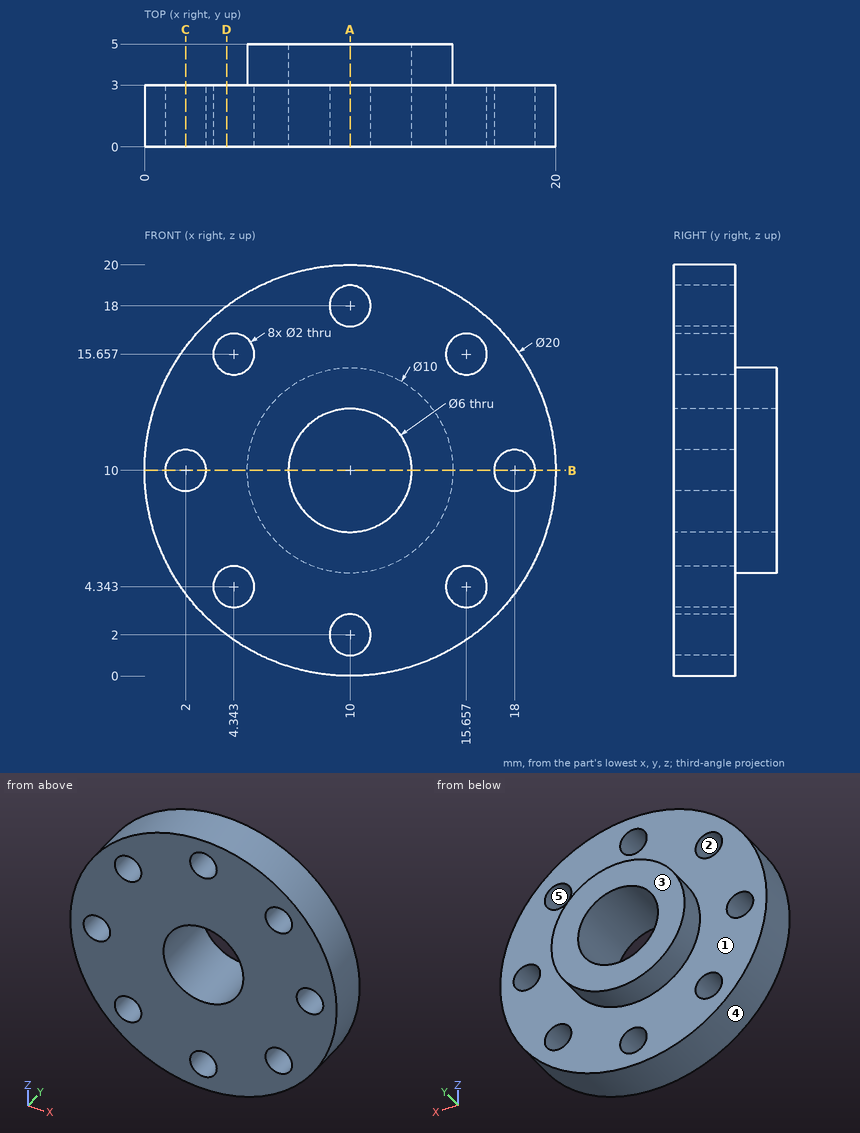
Print and shaded views of the part. All mm, measured from the part's lowest x, y and z. A direction names the side the tool comes from. Coordinates: 2 decimals unless noted, no trailing zeros. Loops run counter-clockwise (first coordinate to the right, second up) from the corner with the lowest first, then second, coordinate; pieces in that order, holes last. Notation, with made-up numbers: (4, -12) - (49, -12) arc R24 cw to (49, 14) - close; hole circle Ø1 at (-24.5, -3). An arc over 180 degrees is marked (long way). Use one line per item in the form item = value. Start each with the question number.
1) Band-saw the part on B-B (z = 10). Give the cut face in (x, y).
2) Drill centre lines: L1, parallel to Z at x = 10, y = 4.15; L2, parallel to X at y = 2.4, z = 5; L3, parallel to Z at x = 10, y = 1. Where is each one in solid material? Low to high. Write a range as from..to.
3) Tool access for the marked faces 1 and 2: list every direction of +Z, -Z, +X, -X, +Y, -Y with a clear straight run to the whole face (end or side of a thin tool).
4) Band-saw the part on D-D (x = 4). Give the cut face in (y, z), and give its area (3 significant figures).
5) Two-plate mould, pull along Z, no slides. Class the marked faces 3, 4 and 5: +Z half, -Z half, draft (parallel to the pull), parting line (faces both ways), or undercut.
6) Flat gauge pins, fed straight in: pin 1 (4 mm diameter, centred on x = 16.5, z = 6, fed in from +Y); pin 2 (3 mm diameter, centred on x = 13, y = 2, fed in from -Z); pin 3 (3 mm diameter, centred on y = 1.5, z = 18, fed in from -X). Where does each tip first touch, or does it go through?
7) Band-saw the part on C-C (x = 2). Give the cut face in (y, z).
8) Band-saw the part on A-A (x = 10). Give the cut face in (y, z), and give its area (3 significant figures).
Check values:
q1.outline = (0, 0) - (1, 0) - (1, 3) - (0, 3) - close; (3, 0) - (7, 0) - (7, 5) - (5, 5) - (5, 3) - (3, 3) - close; (13, 0) - (17, 0) - (17, 3) - (15, 3) - (15, 5) - (13, 5) - close; (19, 0) - (20, 0) - (20, 3) - (19, 3) - close
q2.L1 = 5..7, 13..15
q2.L2 = 1.34..3.59, 5.1..14.9, 16.41..18.66
q2.L3 = 0..1, 3..7, 13..17, 19..20
q3.face_1 = +Y
q3.face_2 = +Y, -Y
q4.outline = (0, 2) - (3, 2) - (3, 3.4) - (0, 3.4) - close; (0, 5.28) - (3, 5.28) - (3, 14.72) - (0, 14.72) - close; (0, 16.6) - (3, 16.6) - (3, 18) - (0, 18) - close
q4.area = 36.7 mm2
q5.face_3 = draft
q5.face_4 = parting line
q5.face_5 = undercut
q6.pin_1 = 3
q6.pin_2 = 0.11
q6.pin_3 = 2.4
q7.outline = (0, 4) - (3, 4) - (3, 9) - (0, 9) - close; (0, 11) - (3, 11) - (3, 16) - (0, 16) - close
q8.outline = (0, 0) - (3, 0) - (3, 1) - (0, 1) - close; (0, 3) - (3, 3) - (3, 5) - (5, 5) - (5, 7) - (0, 7) - close; (0, 13) - (5, 13) - (5, 15) - (3, 15) - (3, 17) - (0, 17) - close; (0, 19) - (3, 19) - (3, 20) - (0, 20) - close
q8.area = 38.0 mm2
